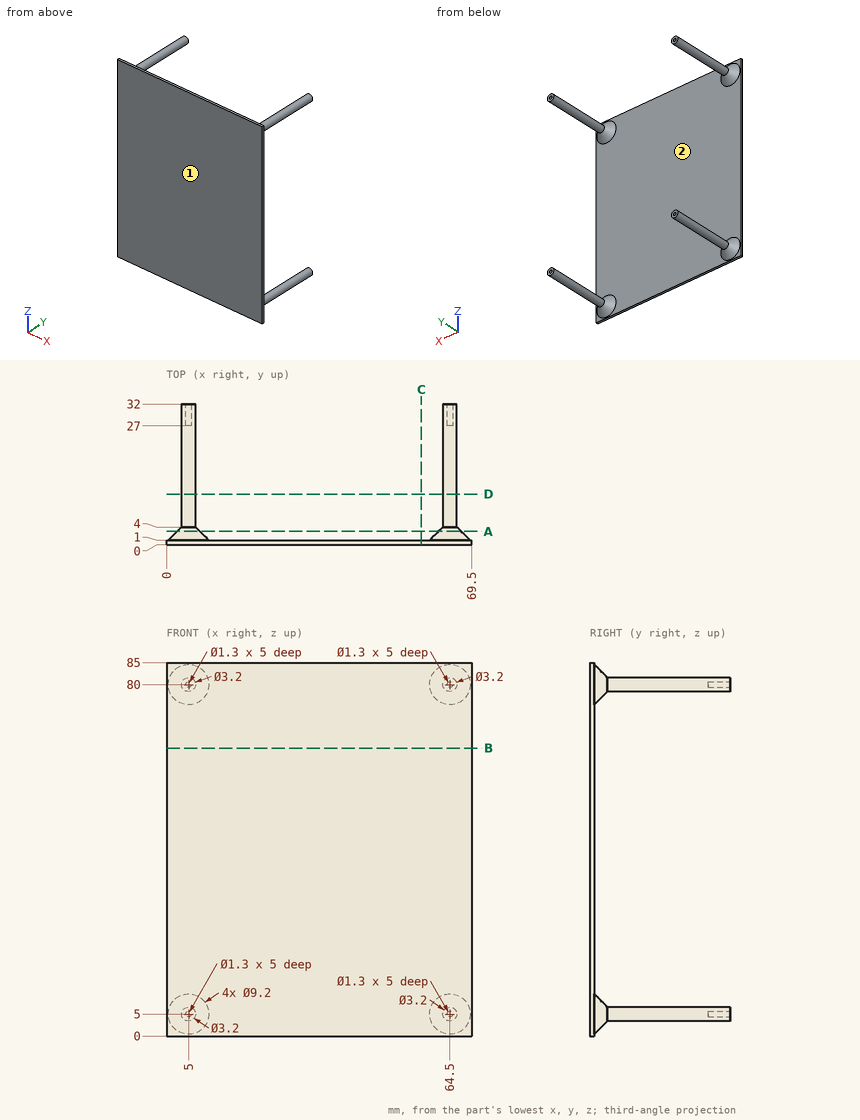
For this review, use the dimensioned drawing (mm, ordinates from the lowest corner) and the shaded views. Coordinates: 2 decimals unless noted, no trailing zeros. Order: outer loops, then holes, each group sorted by start corner. A loop starts at its lowest first (then second) coordinate and runs counter-clockwise, first axis right, second up. Notation, with made-up numbers: (30, -33.75) - (38, -33.75) arc R15 cw to (38, -12.75) - close; hole circle Ø10 at (-19, -10.5). An arc over 180 degrees is marked (long way). Answer in a Markdown table with one row per item.
(1) Consider section B-B on z = 65.5. State the section outline as (x, y) points, plus the area to 3 significant figures.
Checked values:
| item | result |
|---|---|
| outline | (0, 0) - (69.5, 0) - (69.5, 1) - (0, 1) - close |
| area | 69.5 mm^2 |
(2) The part is to be moulded in two halves that separate along X. For the marked faces 1 and 2, say which applies: released by +X, released by -X, zero draft, split by the parting line, or undercut.
Checked values:
| item | result |
|---|---|
| face 1 | zero draft |
| face 2 | undercut |
(3) Clearance check with flat-ended pins moving along their axes: pin 1 (1.2 mm diameter, centred on x = 64.5, z = 80, fed in from +Y); pin 2 (1 mm diameter, centred on x = 35, z = 68.5, fed in from +Y). State where each tip first meets the part, or that it passes through.
Checked values:
| item | result |
|---|---|
| pin 1 | y = 27 |
| pin 2 | y = 1 |
(4) Wall thickness on line 1 along Z through (x, y) = (64.5, 29.8); line 2 along X through (y, z) = (30.85, 80); line 3 along Y through (x, z) = (39, 32.5): over which ranges is each line inside the solid? List them lowest first. Write a range as from..to.
Checked values:
| item | result |
|---|---|
| line 1 | 3.4..4.35, 5.65..6.6, 78.4..79.35, 80.65..81.6 |
| line 2 | 3.4..4.35, 5.65..6.6, 62.9..63.85, 65.15..66.1 |
| line 3 | 0..1 |
(5) Consider section C-C on x = 58. State the section outline as (y, z) points.
Checked values:
| item | result |
|---|---|
| outline | (0, 0) - (1, 0) - (1, 85) - (0, 85) - close |
(6) Consider section A-A on y = 3. State the section outline as (x, z) points, plus the area to 3 significant figures.
Checked values:
| item | result |
|---|---|
| outline | circle Ø5.2 at (5, 5); circle Ø5.2 at (5, 80); circle Ø5.2 at (64.5, 5); circle Ø5.2 at (64.5, 80) |
| area | 84.9 mm^2 |
(7) Consider section D-D on y = 11.5. State the section outline as (x, z) points, plus the area to 3 significant figures.
Checked values:
| item | result |
|---|---|
| outline | circle Ø3.2 at (5, 5); circle Ø3.2 at (5, 80); circle Ø3.2 at (64.5, 5); circle Ø3.2 at (64.5, 80) |
| area | 32.2 mm^2 |
